```python
from build123d import *

# Parameters (mm, degrees)
SKETCH_1_R            = 1.15
SKETCH_1_R_2          = 0.939967297
SKETCH_1_R_3          = 0.967686678
SKETCH_1_R_4          = 1.65
SKETCH_1_W            = 30.4982
SKETCH_1_H            = 42.7098
SKETCH_1_W_2          = 3
SKETCH_1_H_2          = 24
PIXHAWK_M3_DEPTH      = 1.5
SKETCH_2_R            = 1.65
CUT_EXTRUDE_515_DEPTH = 1.5


with BuildPart() as part:
    # 草图1 → Pixhawk正装减振托板_绑带槽_四M3孔 (new body)
    with BuildSketch(Plane.XY):
        Polygon((24, -39), (24, -43), (18, -49), (-18, -49), (-24, -43), (-24, -39), (-30, -33), (-30, 33), (-24, 39), (-24, 43), (-18, 49), (18, 49), (24, 43), (24, 39), (30, 33), (30, -33), align=None)
        with Locations((16, 30)):
            Circle(SKETCH_1_R, mode=Mode.SUBTRACT)
        with Locations((-16, -30)):
            Circle(SKETCH_1_R, mode=Mode.SUBTRACT)
        with Locations((16, -30)):
            Circle(SKETCH_1_R_2, mode=Mode.SUBTRACT)
        with Locations((-16, 30)):
            Circle(SKETCH_1_R_3, mode=Mode.SUBTRACT)
        with Locations((-27, -30)):
            Circle(SKETCH_1_R_4, mode=Mode.SUBTRACT)
        with Locations((-27, 30)):
            Circle(SKETCH_1_R_4, mode=Mode.SUBTRACT)
        with Locations((27, -30)):
            Circle(SKETCH_1_R_4, mode=Mode.SUBTRACT)
        with Locations((27, 30)):
            Circle(SKETCH_1_R_4, mode=Mode.SUBTRACT)
        Rectangle(SKETCH_1_W, SKETCH_1_H, mode=Mode.SUBTRACT)
        with Locations((-26, 0)):
            Rectangle(SKETCH_1_W_2, SKETCH_1_H_2, mode=Mode.SUBTRACT)
        with Locations((26, 0)):
            Rectangle(SKETCH_1_W_2, SKETCH_1_H_2, mode=Mode.SUBTRACT)
    extrude(amount=PIXHAWK_M3_DEPTH)

    # 草图2 → Cut-Extrude 515 (cut)
    with BuildSketch(Plane.XY):
        with Locations((-25, -23)):
            Circle(SKETCH_2_R)
        with Locations((-25, 23)):
            Circle(SKETCH_2_R)
        with Locations((25, -23)):
            Circle(SKETCH_2_R)
        with Locations((25, 23)):
            Circle(SKETCH_2_R)
    extrude(amount=CUT_EXTRUDE_515_DEPTH, mode=Mode.SUBTRACT)


solid = part.part
```
For this review, take the finished solid that the model builds, in its own axes (mm). Coordinates: 2 decimals unless noted, no trailing zeros. Order: outer loops, then holes, each group sorted by start corner. A loop starts at its lowest first (then second) coordinate and runs counter-clockwise, first axis right, second up. Notation, with made-up numbers: (22, -30) -> (28, -30) arc R10 ccw to (28, -20) -> close; hole circle Ø2 at (-40, 57.25). An arc over 180 degrees is marked (long way). Use CSV: the item, a comma, the result in double quotes. Start each with the question number.
Item 1: We need section C-C, the plane y = 23. Give the boundary of the cut face in (x, z).
Item 2: We need section B-B, the plane y = -30. Give the boundary of the cut face in (x, z), then the cut area to 3 significant figures.
Item 3: Draft analysis for pull direction Y (two halves, no side actions). For faces 1 (the face through (27, -36, 1)), 2 (the face through (25.784, -28.885, 0.74)), 3 (the face through (20, 1, 0)), state which applies: pulls with the +Y half, pulls with the -Y half, needs draft (parallel to the pull), parting line crosses it, or undercut.
Item 4: We need section D-D, the plane z = 0.8. Give the number of separate pieces and of enclosed holes in the cut face, then the cut area to 3 significant figures.
Item 5: Wall thickness on probe 1 along Y at (x, z) = (16, 0.4); probe 2 along X at (y, z) = (-7.5, 1.4); probe 3 along Y at (x, z) = (8, 0.65): over which ranges is each line inside the solid? List them lowest first.
Item 6: We need section A-A, the plane x = 13.5. Give the boundary of the cut face in (y, z).
Item 7: Insertion check: pin 1 (0.8 mm diameter, centred on y = 42, z = 1, fed in from -X); pin 2 (10 mm diameter, centred on x = -4.5, y = -16.5, fed in from -Z); pin 3 (0.8 mm diameter, centred on x = -26, z = 1, fed in from +Y). Each pin has a flat end and moves straight along its axis. Give the tip position at first contact, or say it passes through.
Derived:
1,outline,"(-30, 0) -> (-26.65, 0) -> (-26.65, 1.5) -> (-30, 1.5) -> close; (-23.35, 0) -> (23.35, 0) -> (23.35, 1.5) -> (-23.35, 1.5) -> close; (26.65, 0) -> (30, 0) -> (30, 1.5) -> (26.65, 1.5) -> close"
2,outline,"(-30, 0) -> (-28.65, 0) -> (-28.65, 1.5) -> (-30, 1.5) -> close; (-25.35, 0) -> (-17.15, 0) -> (-17.15, 1.5) -> (-25.35, 1.5) -> close; (-14.85, 0) -> (15.06, 0) -> (15.06, 1.5) -> (-14.85, 1.5) -> close; (16.94, 0) -> (25.35, 0) -> (25.35, 1.5) -> (16.94, 1.5) -> close; (28.65, 0) -> (30, 0) -> (30, 1.5) -> (28.65, 1.5) -> close"
2,area,"73.8 mm^2"
3,face 1,"pulls with the -Y half"
3,face 2,"undercut"
3,face 3,"needs draft"
4,separate pieces,"1"
4,enclosed holes,"15"
4,area,"3,970 mm^2"
5,probe 1,"y = -49 to -30.94, -29.06 to 28.85, 31.15 to 49"
5,probe 2,"x = -30 to -27.5, -24.5 to -15.25, 15.25 to 24.5, 27.5 to 30"
5,probe 3,"y = -49 to -21.35, 21.35 to 49"
6,outline,"(-49, 0) -> (-21.35, 0) -> (-21.35, 1.5) -> (-49, 1.5) -> close; (21.35, 0) -> (49, 0) -> (49, 1.5) -> (21.35, 1.5) -> close"
7,pin 1,"stops at x = -24"
7,pin 2,"stops at z = 0"
7,pin 3,"stops at y = 37.4"
